Geometry check sheet. Reference: the model listing, model coordinates, mm. A direction names the side the tool comes from. Coordinates: 2 decimals unless noted, no trailing zeros. Loops run counter-clockwise (first coordinate to the right, second up) from the corner with the lowest first, then second, coordinate; pieces in that order, holes last. Notation, with made-up numbers: (-21.5, 21.5) - (34.5, 21.5) arc R14 ccw to (34.5, 25.5) - close; hole circle Ø11 at (-3.5, 11.5). An arc over 180 degrees is marked (long way). One line per item, written item: value.
Autodesk Fusion 360 part; units mm, degrees
sketch "Sketch1" plane through (0, 0, 0) normal (0, 0, 1) x (1, 0, 0)
  circle A0 centre (0, 45) radius 1.75
  circle A1 centre (50, 45) radius 1.75
  circle A2 centre (0, 0) radius 1.75
  circle A3 centre (50, 0) radius 1.75
  line L0 (54, 45) -> (54, 0)
  line L1 (-4, 0) -> (-4, 45)
  line L2 (0, 49) -> (50, 49)
  line L3 (50, -4) -> (0, -4)
  line L4 (-1.75, 45) -> (1.75, 45)
  line L5 (48.25, 45) -> (51.75, 45)
  line L6 (50, 45) -> (48.25, 45)
  line L7 (1.75, 45) -> (0, 45)
  line L8 (0, -1.75) -> (0, 1.75)
  line L9 (0, 43.25) -> (0, 46.75)
  line L10 (0, 45) -> (0, 43.25)
  line L11 (0, 1.75) -> (0, 0)
  arc A4 (0, 49) -> (-4, 44.9977) centre (0, 45) ccw
  line L12 (50, 46.75) -> (50, 43.25)
  line L13 (50, 1.75) -> (50, -1.75)
  line L14 (50, 0) -> (50, 1.75)
  line L15 (50, 43.25) -> (50, 45)
  arc A5 (54, 45) -> (50, 49) centre (50, 45) ccw
  arc A6 (50, -4) -> (54, 0) centre (50, 0) ccw
  line L16 (0, 0) -> (1.75, 0)
  line L17 (48.25, 0) -> (50, 0)
  line L18 (51.75, 0) -> (48.25, 0)
  line L19 (1.75, 0) -> (-1.75, 0)
  arc A7 (-4, 0) -> (0, -4) centre (0, 0) ccw
  circle A8 centre (0, 0) radius 2.5
  circle A9 centre (0, 45) radius 2.5
  circle A10 centre (50, 45) radius 2.5
  circle A11 centre (50, 0) radius 2.5
  line L20 (0, 0) -> (5, 0)
  line L21 (5, 0) -> (5, 5)
  line L22 (5, 5) -> (0, 5)
  line L23 (0, 5) -> (0, 0)
  circle A12 centre (5, 5) radius 2.625
  dimension "d1" = 50
  dimension "d2" = 45
  dimension "d3" = 3.5
  dimension "d4" = 3.5
  dimension "d5" = 3.5
  dimension "d6" = 3.5
  dimension "d7" = 8
  dimension "d9" = 8
  dimension "d10" = 8
  dimension "d11" = 5
  dimension "d12" = 5
  dimension "d13" = 5
  dimension "d14" = 5
  dimension "d19" = 5
  dimension "d20" = 5.25
extrude "Extrude1" add sketch "Sketch1" along normal blind 2 contours A8 L20 L21 L22 L23 A12 | L21 L22 A12 | L21 L22 A12 | L0 L1 L2 L3 A4 A5 A6 A7
extrude "Extrude2" add sketch "Sketch1" along normal blind 4.5 contours A2 A8 L20 L23 | A2 A8 L20 L23 | A9 | A10 | A11
extrude "Extrude3" cut sketch "Sketch1" along normal blind 10 contours L21 L22 A12 | L21 L22 A12
(1) Cross-section at B-B on y = 5. Record the cut outline in (x, z) (3 decimals).
Reply:
outline: (-4, 0) - (2.375, 0) - (2.375, 2) - (-4, 2) - close; (7.625, 0) - (54, 0) - (54, 2) - (7.625, 2) - close
(2) Go/stop test with a flat-tipped pin: pin 1 Ø16 at (x, y) = (39.5, 19.5) entering from +Z. Record where the tip stops, or that it passes through.
Reply:
pin 1: z = 2
(3) Release check for a two-part mould opening along X. For faces 1 (the face through (52.31, 45.96, 3.23)), 2 (the face through (52.859, -2.797, 0.986)), 3 (the face through (-2.797, -2.859, 0.986)), 4 (the face through (25, -4, 1)) record: pulls with the +X half, pulls with the -X half, needs draft (parallel to the pull), parting line crosses it, or undercut.
Reply:
face 1: undercut
face 2: pulls with the +X half
face 3: pulls with the -X half
face 4: needs draft
(4) Cross-section at C-C on x = 5. Record the cut outline in (y, z) (3 decimals).
Reply:
outline: (-4, 0) - (2.375, 0) - (2.375, 2) - (-4, 2) - close; (7.625, 0) - (49, 0) - (49, 2) - (7.625, 2) - close
(5) Cross-section at D-D on x = 37. Record the cut outline in (y, z).
Reply:
outline: (-4, 0) - (49, 0) - (49, 2) - (-4, 2) - close
(6) Access from +Z, -Z, +X, -X, +Y, -Y to the whole of each face (thin tool, end or side, straight path). Record for faces 5 (the face through (1.617, 0.67, 2.218)), 6 (the face through (-0.54, 47.44, 3.23)).
Reply:
face 5: +Z, -Z
face 6: +Z
(7) Material ranges on probe 1 along X at (y, z) = (45, 1.7); probe 2 along Y at (x, z) = (50, 0.8); probe 3 along X at (y, z) = (5, 0.7) (3 decimals), recorded low to high. Write a range as from..to.
Reply:
probe 1: -4..-1.75, 1.75..48.25, 51.75..54
probe 2: -4..-1.75, 1.75..43.25, 46.75..49
probe 3: -4..2.375, 7.625..54
(8) Cross-section at A-A on z = 3.4. Record the cut outline in (x, y), and give its area (3 significant figures).
Reply:
outline: circle Ø5 at (0, 0); circle Ø5 at (0, 45); circle Ø5 at (50, 0); circle Ø5 at (50, 45); hole circle Ø3.5 at (0, 0); hole circle Ø3.5 at (0, 45); hole circle Ø3.5 at (50, 0); hole circle Ø3.5 at (50, 45)
area: 40.1 mm2
